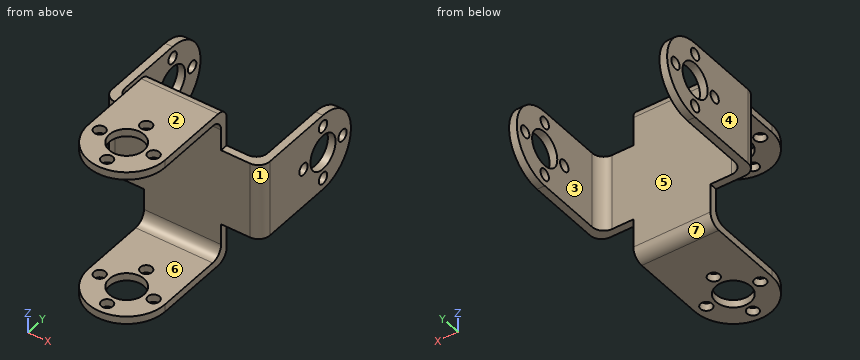
from build123d import *

# Parameters (mm, degrees)
EXTRUDE_1_DEPTH     = 2
SKETCH_2_W          = 2
SKETCH_2_H          = 20
EXTRUDE_2_DEPTH     = 40
FILLET_1_R          = 3
SKETCH_4_W          = 20
SKETCH_4_H          = 2
EXTRUDE_3_DEPTH     = 40
FILLET_2_R          = 3
SKETCH_5_R          = 4.5
SKETCH_5_R_2        = 1.5
CUT_EXTRUDE_1_DEPTH = 63.171134781
SKETCH_6_R          = 4.5
SKETCH_6_R_2        = 1.5
CUT_EXTRUDE_2_DEPTH = 63.171134781


with BuildPart() as part:
    # 草图1 → 凸台-拉伸1 (new body)
    with BuildSketch(Plane(origin=(0, 0, 0), x_dir=(1, 0, 0), z_dir=(0, 1, 0))):
        Polygon((10, -10), (10, -20.5), (-10, -20.5), (-10, -10), (-20.5, -10), (-20.5, 10), (-10, 10), (-10, 20.5), (10, 20.5), (10, 10), (20.5, 10), (20.5, -10), align=None)
    extrude(amount=EXTRUDE_1_DEPTH)

    # 草图2 → 凸台-拉伸2 (add)
    with BuildSketch(Plane(origin=(0, 2, 0), x_dir=(1, 0, 0), z_dir=(0, 1, 0))):
        with Locations((-19.5, 0)):
            Rectangle(SKETCH_2_W, SKETCH_2_H)
        with Locations((19.5, 0)):
            Rectangle(SKETCH_2_W, SKETCH_2_H)
    extrude(amount=EXTRUDE_2_DEPTH)

    # 圆角1
    fillet_1_edges = [part.edges().sort_by_distance(p)[0] for p in [
        (-20.5, 0, 0),
        (20.5, 0, 0),
        (-18.5, 2, 0),
        (18.5, 2, 0),
    ]]
    fillet(fillet_1_edges, radius=FILLET_1_R)

    # 草图4 → 凸台-拉伸3 (add)
    with BuildSketch(Plane.XZ):
        with Locations((0, 19.5)):
            Rectangle(SKETCH_4_W, SKETCH_4_H)
        with Locations((0, -19.5)):
            Rectangle(SKETCH_4_W, SKETCH_4_H)
    extrude(amount=EXTRUDE_3_DEPTH)

    # 圆角2
    fillet_2_edges = [part.edges().sort_by_distance(p)[0] for p in [
        (0, 2, -20.5),
        (0, 2, 20.5),
        (0, 0, 18.5),
        (0, 0, -18.5),
    ]]
    fillet(fillet_2_edges, radius=FILLET_2_R)

    # 草图5 → 切除-拉伸1 (cut, through all)
    with BuildSketch(Plane(origin=(0, 0, -20.5), x_dir=(-1, 0, 0), z_dir=(0, 0, -1))):
        with Locations((0, -20)):
            Circle(SKETCH_5_R)
        with Locations((0, -13)):
            Circle(SKETCH_5_R_2)
        with Locations((7, -20)):
            Circle(SKETCH_5_R_2)
        with Locations((0, -27)):
            Circle(SKETCH_5_R_2)
        with Locations((-7, -20)):
            Circle(SKETCH_5_R_2)
        with BuildLine():
            Line((-10, -20), (-10, -40))
            Line((-10, -40), (10, -40))
            Line((10, -40), (10, -20))
            ThreePointArc((10, -20), (0, -30), (-10, -20))
        make_face()
    extrude(amount=-CUT_EXTRUDE_1_DEPTH, mode=Mode.SUBTRACT)

    # 草图6 → 切除-拉伸2 (cut, through all)
    with BuildSketch(Plane.ZY.offset(20.5)):
        with Locations((0, 22)):
            Circle(SKETCH_6_R)
        with Locations((0, 15)):
            Circle(SKETCH_6_R_2)
        with Locations((-7, 22)):
            Circle(SKETCH_6_R_2)
        with Locations((0, 29)):
            Circle(SKETCH_6_R_2)
        with Locations((7, 22)):
            Circle(SKETCH_6_R_2)
        with BuildLine():
            Line((-10, 22), (-10, 42))
            Line((-10, 42), (10, 42))
            Line((10, 42), (10, 22))
            ThreePointArc((10, 22), (0, 32), (-10, 22))
        make_face()
    extrude(amount=-CUT_EXTRUDE_2_DEPTH, mode=Mode.SUBTRACT)


solid = part.part
Geometry check sheet. Reference: the model listing, model coordinates, mm. Face numbers are marked on the shaded views. A direction names the side the tool comes from. Give positions to 0.01 mm unless a question says otherwise; leave off trailing zeros. Loops run counter-clockwise (first coordinate to the right, second up) from the corner with the lowest first, then second, coordinate; pieces in that order, holes last.
(1) Section check D-D on z = -7. Record the cut outline in (x, y), then the cut area to 3 significant figures.
From the geometry:
outline: (-20.5, 3) arc R3 ccw to (-17.5, 0) - (17.5, 0) arc R3 ccw to (20.5, 3) - (20.5, 20.5) - (18.5, 20.5) - (18.5, 5) arc R3 cw to (15.5, 2) - (-15.5, 2) arc R3 cw to (-18.5, 5) - (-18.5, 20.5) - (-20.5, 20.5) - close; (-20.5, 23.5) - (-18.5, 23.5) - (-18.5, 29.14) - (-20.5, 29.14) - close; (18.5, 23.5) - (20.5, 23.5) - (20.5, 29.14) - (18.5, 29.14) - close
area: 179 mm2
(2) Depth check by flat-ended pin: pin 1 Ø2.5 at (y, z) = (22, 7) entering from +X; pin 2 Ø15.5 at (x, z) = (-5, 5.5) entering from -Y; pin 3 Ø3 at (x, z) = (-7.5, 0.5) entering from +Y; pin 4 Ø4 at (x, y) = (-8.5, 1.5) entering from +Z. Enter the tip coordinate at first touch or a pass-through.
From the geometry:
pin 1: passes through
pin 2: stops at y = 0
pin 3: stops at y = 2
pin 4: stops at z = 20.46
(3) Release check for a two-part mould opening along X. For the marked faces 1, 2, 3 and 4 record: released by +X, released by -X, zero draft, split by the parting line, or undercut.
From the geometry:
face 1: released by +X
face 2: zero draft
face 3: undercut
face 4: released by -X
(4) Thickness scan on L1, parallel to Y at x = 20, z = 0; L2, parallel to Z at x = 4.5, y = -7; L3, parallel to Y at x = 0, z = -19. Record the ranges inside material, lowest first.
From the geometry:
L1: y = 1.34 to 13.5, 16.5 to 17.5, 26.5 to 27.5, 30.5 to 32
L2: z = -20.5 to -18.5, 18.5 to 20.5
L3: y = -30 to -28.5, -25.5 to -24.5, -15.5 to -14.5, -11.5 to 1.6
(5) Section check B-B on y = 15. Record the cut outline in (x, z), then the cut area to 3 significant figures.
From the geometry:
outline: (-20.5, -10) - (-18.5, -10) - (-18.5, -1.5) - (-20.5, -1.5) - close; (-20.5, 1.5) - (-18.5, 1.5) - (-18.5, 10) - (-20.5, 10) - close; (18.5, -10) - (20.5, -10) - (20.5, -1.5) - (18.5, -1.5) - close; (18.5, 1.5) - (20.5, 1.5) - (20.5, 10) - (18.5, 10) - close
area: 68.0 mm2
(6) Section check A-A on y = -5.5. Record the cut outline in (x, z), then the cut area to 3 significant figures.
From the geometry:
outline: (-10, -20.5) - (10, -20.5) - (10, -18.5) - (-10, -18.5) - close; (-10, 18.5) - (10, 18.5) - (10, 20.5) - (-10, 20.5) - close
area: 80.0 mm2
(7) Set-up check for the marked faces 5, 6 and 7: record each of +Z, -Z, +X, -X, +Y, -Y from which the full face is reachable in a straight line by a thin tool's end or side.
From the geometry:
face 5: +Z, -Z, +Y
face 6: +X, -X, -Y
face 7: -Z, +X, -X, +Y
(8) Section check C-C on x = -7. Record the cut outline in (y, z).
From the geometry:
outline: (-27.14, -20.5) - (-21.5, -20.5) - (-21.5, -18.5) - (-27.14, -18.5) - close; (-27.14, 18.5) - (-21.5, 18.5) - (-21.5, 20.5) - (-27.14, 20.5) - close; (-18.5, -20.5) - (-1, -20.5) arc R3 ccw to (2, -17.5) - (2, 17.5) arc R3 ccw to (-1, 20.5) - (-18.5, 20.5) - (-18.5, 18.5) - (-3, 18.5) arc R3 cw to (0, 15.5) - (0, -15.5) arc R3 cw to (-3, -18.5) - (-18.5, -18.5) - close
